CAD build for the part. Positions are in the model's coordinates, mm. A direction names the side the tool comes from. Give positions to 0.01 mm unless a question says otherwise; leave off trailing zeros. Write each loop counter-clockwise with the first axis right and the second up, starting at its lowest first coordinate (ties: lowest second). Pieces come first, ordered by that corner, then holes. Notation, with made-up numbers: (85.25, 25) - (95.25, 25) arc R18 cw to (95.25, 51) - close; hole circle Ø11 at (-31.5, -24). An arc over 180 degrees is marked (long way). Answer as a JSON object with one key per item and string values.
from build123d import *

# Parameters (mm, degrees)
SALIENTE_EXTRUIR1_DEPTH    = 40
CROQUIS2_W                 = 20
CROQUIS2_H                 = 13
SALIENTE_EXTRUIR2_DEPTH    = 10
CROQUIS3_R                 = 2.125
CORTAR_EXTRUIR1_DEPTH      = 56.398555938
CORTAR_EXTRUIR2_DEPTH      = 56.398555938
CORTAR_EXTRUIR2_DEPTH_BACK = 5
CROQUIS4_R                 = 4.05
CORTAR_EXTRUIR3_DEPTH      = 56.398555938
CORTAR_EXTRUIR3_DEPTH_BACK = 56.398555938
CROQUIS5_R                 = 2.125
CORTAR_EXTRUIR4_DEPTH      = 58.445626465
CORTAR_EXTRUIR4_DEPTH_BACK = 5
CORTAR_EXTRUIR4_START      = -7
CROQUIS6_R                 = 4.05
CORTAR_EXTRUIR5_START      = -7
CORTAR_EXTRUIR5_DEPTH      = 7
CORTAR_EXTRUIR6_DEPTH      = 7
CROQUIS9_R                 = 2.125
CORTAR_EXTRUIR7_DEPTH      = 58.445626465
CORTAR_EXTRUIR8_DEPTH      = 58.445626465
CORTAR_EXTRUIR8_DEPTH_BACK = 5
CORTAR_EXTRUIR8_START      = -7
CROQUIS10_R                = 4.05


with BuildPart() as part:
    # Croquis1 → Saliente-Extruir1 (new body)
    with BuildSketch(Plane(origin=(0, 0, 0), x_dir=(1, 0, 0), z_dir=(0, 1, 0))):
        Polygon((0, 0), (0, 20), (20, 20), (20, 7), (13, 7), (13, 0), align=None)
    extrude(amount=SALIENTE_EXTRUIR1_DEPTH)

    # Croquis2 → Saliente-Extruir2 (add)
    with BuildSketch(Plane(origin=(0, 40, 0), x_dir=(1, 0, 0), z_dir=(0, 1, 0))):
        with Locations((10, 13.5)):
            Rectangle(CROQUIS2_W, CROQUIS2_H)
    extrude(amount=SALIENTE_EXTRUIR2_DEPTH)

    # Croquis3 → Cortar-Extruir1 (cut, through all)
    with BuildSketch(Plane(origin=(13, 0, 0), x_dir=(0, 0, -1), z_dir=(1, 0, 0))):
        with Locations((10, 30)):
            Circle(CROQUIS3_R)
        with Locations((10, 10)):
            Circle(CROQUIS3_R)
    extrude(amount=-CORTAR_EXTRUIR1_DEPTH, mode=Mode.SUBTRACT)

    # Croquis4 → Cortar-Extruir2 (cut, two sides: drawn at the far end of the back side and taken through both)
    with BuildSketch(Plane(origin=(13, 0, 0), x_dir=(0, 0, -1), z_dir=(1, 0, 0)).offset(-CORTAR_EXTRUIR2_DEPTH_BACK)):
        with Locations(Location((10, 30, 0), (0, 0, 222.205446404))):
            Circle(CROQUIS4_R)
        with Locations(Location((10, 10, 0), (0, 0, 222.205446404))):
            Circle(CROQUIS4_R)
    extrude(amount=CORTAR_EXTRUIR2_DEPTH + CORTAR_EXTRUIR2_DEPTH_BACK, mode=Mode.SUBTRACT)

    # Croquis5 → Cortar-Extruir3 (cut, two sides: drawn at the far end of the back side and taken through both)
    with BuildSketch(Plane.XY.offset(-7).offset(-CORTAR_EXTRUIR3_DEPTH_BACK)):
        with Locations((10, 20)):
            Circle(CROQUIS5_R)
    extrude(amount=CORTAR_EXTRUIR3_DEPTH + CORTAR_EXTRUIR3_DEPTH_BACK, mode=Mode.SUBTRACT)

    # Croquis6 → Cortar-Extruir4 (cut, two sides: drawn at the far end of the back side and taken through both)
    with BuildSketch(Plane.XY.offset(CORTAR_EXTRUIR4_START - CORTAR_EXTRUIR4_DEPTH_BACK)):
        with Locations(Location((10, 20, 0), (0, 0, 180))):
            Circle(CROQUIS6_R)
    extrude(amount=CORTAR_EXTRUIR4_DEPTH + CORTAR_EXTRUIR4_DEPTH_BACK, mode=Mode.SUBTRACT)

    # Croquis7 → Cortar-Extruir5 (cut)
    with BuildSketch(Plane.XY.offset(CORTAR_EXTRUIR5_START)):
        with BuildLine():
            Line((10, 24.05), (18, 24.05))
            Line((18, 24.05), (18, 15.95))
            Line((18, 15.95), (10, 15.95))
            ThreePointArc((10, 15.95), (14.05, 20), (10, 24.05))
        make_face()
    extrude(amount=CORTAR_EXTRUIR5_DEPTH, mode=Mode.SUBTRACT)

    # Croquis8 → Cortar-Extruir6 (cut)
    with BuildSketch(Plane(origin=(20, 0, 0), x_dir=(0, 0, -1), z_dir=(1, 0, 0))):
        with BuildLine():
            Line((10, 34.05), (0, 34.05))
            Line((0, 34.05), (0, 25.95))
            Line((0, 25.95), (10, 25.95))
            ThreePointArc((10, 25.95), (5.95, 30), (10, 34.05))
        make_face()
        with BuildLine():
            Line((10, 14.05), (0, 14.05))
            Line((0, 14.05), (0, 5.95))
            Line((0, 5.95), (10, 5.95))
            ThreePointArc((10, 5.95), (5.95, 10), (10, 14.05))
        make_face()
    extrude(amount=-CORTAR_EXTRUIR6_DEPTH, mode=Mode.SUBTRACT)

    # Croquis9 → Cortar-Extruir7 (cut, through all)
    with BuildSketch(Plane.XY):
        with Locations((10, 40)):
            Circle(CROQUIS9_R)
    extrude(amount=-CORTAR_EXTRUIR7_DEPTH, mode=Mode.SUBTRACT)

    # Croquis10 → Cortar-Extruir8 (cut, two sides: drawn at the far end of the back side and taken through both)
    with BuildSketch(Plane.XY.offset(CORTAR_EXTRUIR8_START - CORTAR_EXTRUIR8_DEPTH_BACK)):
        with Locations(Location((10, 40, 0), (0, 0, 180))):
            Circle(CROQUIS10_R)
    extrude(amount=CORTAR_EXTRUIR8_DEPTH + CORTAR_EXTRUIR8_DEPTH_BACK, mode=Mode.SUBTRACT)


solid = part.part
Item 1: Flat gauge pins, fed straight in: P1, Ø9, axis at y = 11.5, z = -11.5, coming from the +X side; P2, Ø1, axis at x = 2.5, z = -2, coming from the +Y side; P3, Ø7.5, axis at y = 30, z = -10, coming from the +X side; P4, Ø4, axis at x = 10.5, y = 19.5, coming from the +Z side. Where does each tip first touch, or does it go through?
Entries:
{"P1": "x = 20", "P2": "y = 40", "P3": "x = 8", "P4": "z = -12"}
Item 2: Which spindle directions (+Z, -Z, +X, -X, +Y, -Y) get a long thin tool onto all of the face, cutting with end or side? Do faces 1 (the flat face through (8, 22, -12)), 2 (the flat face through (12, 15.95, -4)), 3 (the flat face through (8, 30.1, -7.5)). Say none if no direction does.
Entries:
{"face 1": "+Z", "face 2": "+Z, +X", "face 3": "+X"}
Item 3: Mould opens along Y. For faces 4 (the flat face through (10, 0, -10)), 5 (the cylindrical face through (4.06, 8.71, -8.31)), 6 (the flat face through (16, 3, -7)), 7 (the flat face through (3, 40, -4)) say: +Y half, -Y half, draft (parallel to the pull), parting line (faces both ways), or undercut.
Entries:
{"face 4": "-Y half", "face 5": "undercut", "face 6": "draft", "face 7": "+Y half"}
Item 4: Cut at C-C (x = 2.5). Give the cut face in (y, z) (3 decimals), and give its area (3 significant figures).
Entries:
{"outline": "(0, -20) - (50, -20) - (50, -7) - (40, -7) - (40, 0) - (0, 0) - close; hole circle Ø4.25 at (10, -10); hole circle Ø4.25 at (30, -10)", "area": "902 mm2"}
Item 5: Cut at B-B (y = 20). Give the cut face in (x, z) (3 decimals).
Entries:
{"outline": "(0, -20) - (7.875, -20) - (7.875, -12) - (5.95, -12) - (5.95, 0) - (0, 0) - close; (12.125, -20) - (20, -20) - (20, -7) - (14.05, -7) - (14.05, -12) - (12.125, -12) - close"}
Item 6: Cut at A-A (x = 10.5). State how many separate pieces and enclosed holes the cut face has, and give its area (3 significant figures).
Entries:
{"separate pieces": "3", "enclosed holes": "2", "area": "596 mm2"}
Item 7: Cut at D-D (z = -18.25). Give the cut face in (x, y) (3 decimals).
Entries:
{"outline": "(0, 0) - (20, 0) - (20, 50) - (0, 50) - close; hole circle Ø4.25 at (10, 20); hole circle Ø4.25 at (10, 40)"}
Item 8: Probe line 1 (Y direction, x = 2.5, z = -10) (3 decimals); line 2 (Y direction, x = 10, z = -16.75) (3 decimals); line 3 (Y direction, x = 10, z = -5.5). List the from-to ranges inside material, lowest first. Write a range as from..to.
Entries:
{"line 1": "0..7.875, 12.125..27.875, 32.125..50", "line 2": "0..17.875, 22.125..37.875, 42.125..50", "line 3": "0..15.95, 24.05..35.95"}
